from build123d import *

# Parameters (mm, degrees)
CROQUIS1_R              = 3
CROQUIS1_R_2            = 1
SALIENTE_EXTRUIR1_DEPTH = 5


with BuildPart() as part:
    # Croquis1 → Saliente-Extruir1 (new body)
    with BuildSketch(Plane.XY):
        with BuildLine():
            Line((-20, 0), (-20, 23))
            Line((-20, 23), (20, 23))
            Line((20, 23), (20, 0))
            ThreePointArc((20, 0), (0, -20), (-20, 0))
        make_face()
        with Locations((10, 0)):
            Circle(CROQUIS1_R, mode=Mode.SUBTRACT)
        with Locations((-10, 0)):
            Circle(CROQUIS1_R, mode=Mode.SUBTRACT)
        with Locations((-10, 18)):
            Circle(CROQUIS1_R, mode=Mode.SUBTRACT)
        with Locations((10, 18)):
            Circle(CROQUIS1_R, mode=Mode.SUBTRACT)
        with Locations((-4, 18)):
            Circle(CROQUIS1_R_2, mode=Mode.SUBTRACT)
        with Locations((-16, 18)):
            Circle(CROQUIS1_R_2, mode=Mode.SUBTRACT)
        with Locations((4, 18)):
            Circle(CROQUIS1_R_2, mode=Mode.SUBTRACT)
        with Locations((16, 18)):
            Circle(CROQUIS1_R_2, mode=Mode.SUBTRACT)
    extrude(amount=SALIENTE_EXTRUIR1_DEPTH)


solid = part.part
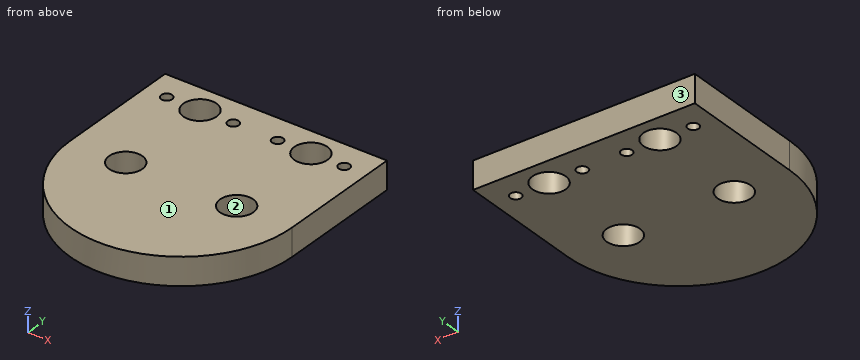
Here's how the part is built. I have some questions about the finished solid (model axes, mm). Face numbers are marked on the shaded views. Coordinates: 2 decimals unless noted, no trailing zeros. Order: outer loops, then holes, each group sorted by start corner. A loop starts at its lowest first (then second) coordinate and runs counter-clockwise, first axis right, second up. Notation, with made-up numbers: (-26.5, 59.25) -> (-0.5, 59.25) arc R8 cw to (-0.5, 63.25) -> close; hole circle Ø4 at (2.25, 24.5). An arc over 180 degrees is marked (long way). Answer in a Markdown table with one row per item.
(1) I want a section at A-A on z = 4.15. Count the separate pieces of the cut face and the enclosed holes in it, then the cut area to 3 significant figures.
Answer key:
| item | result |
|---|---|
| separate pieces | 1 |
| enclosed holes | 8 |
| area | 1,420 mm^2 |
(2) Thinking about a two-plate mould opening in Y: for the marked faces 1, 2 and 3, which applies, +Y half, -Y half, draft (parallel to the pull), parting line (faces both ways), or undercut?
Answer key:
| item | result |
|---|---|
| face 1 | draft |
| face 2 | undercut |
| face 3 | +Y half |
(3) I want a section at C-C on y = 18. List the corners of the cut face in (x, z) for me, then the cut area to 3 significant figures.
Answer key:
| item | result |
|---|---|
| outline | (-20, 0) -> (-17, 0) -> (-17, 5) -> (-20, 5) -> close; (-15, 0) -> (-13, 0) -> (-13, 5) -> (-15, 5) -> close; (-7, 0) -> (-5, 0) -> (-5, 5) -> (-7, 5) -> close; (-3, 0) -> (3, 0) -> (3, 5) -> (-3, 5) -> close; (5, 0) -> (7, 0) -> (7, 5) -> (5, 5) -> close; (13, 0) -> (15, 0) -> (15, 5) -> (13, 5) -> close; (17, 0) -> (20, 0) -> (20, 5) -> (17, 5) -> close |
| area | 100 mm^2 |
(4) Please list where these lines run through material, in increasing order: probe 1 along Y at (x, z) = (8.5, 2.9); probe 2 along Y at (x, z) = (12, 4.7); probe 3 along Y at (x, z) = (-16, 4.2).
Answer key:
| item | result |
|---|---|
| probe 1 | -18.1 to -2.6, 2.6 to 15.4, 20.6 to 23 |
| probe 2 | -16 to -2.24, 2.24 to 15.76, 20.24 to 23 |
| probe 3 | -12 to 17, 19 to 23 |
(5) I want a section at B-B on x = -16. List the corners of the cut face in (y, z) for me.
Answer key:
| item | result |
|---|---|
| outline | (-12, 0) -> (17, 0) -> (17, 5) -> (-12, 5) -> close; (19, 0) -> (23, 0) -> (23, 5) -> (19, 5) -> close |
(6) I want a section at D-D on x = 10. List the corners of the cut face in (y, z) for me, then the cut area to 3 significant figures.
Answer key:
| item | result |
|---|---|
| outline | (-17.32, 0) -> (-3, 0) -> (-3, 5) -> (-17.32, 5) -> close; (3, 0) -> (15, 0) -> (15, 5) -> (3, 5) -> close; (21, 0) -> (23, 0) -> (23, 5) -> (21, 5) -> close |
| area | 142 mm^2 |
(7) Will these pins go through, and if not, where does the flat tip stop? pin 1 Ø7 at (x, y) = (10, 0) entering from +Z; pin 2 Ø3 at (x, z) = (-6.5, 1) entering from -Y.
Answer key:
| item | result |
|---|---|
| pin 1 | z = 5 |
| pin 2 | y = -19.36 |
